from build123d import *

# Parameters (mm, degrees)
SKETCH_R  = 3.302
PAD_DEPTH = 3


with BuildPart() as part:
    # Sketch → Pad (new body)
    with BuildSketch(Plane.XY):
        with BuildLine():
            Line((0, 62.5), (0, 1))
            ThreePointArc((0, 1), (0.292893, 0.292893), (1, 0))
            Line((1, 0), (43.41875, 0))
            ThreePointArc((43.41875, 0), (44.125857, 0.292893), (44.41875, 1))
            Line((44.41875, 1), (44.41875, 24.9))
            ThreePointArc((45.41875, 25.9), (44.711643, 25.607107), (44.41875, 24.9))
            Line((45.41875, 25.9), (125.41865, 25.9))
            ThreePointArc((125.41865, 25.9), (126.125757, 26.192893), (126.41865, 26.9))
            Line((126.41865, 26.9), (126.41865, 62.5))
            ThreePointArc((126.41865, 62.5), (126.125757, 63.207107), (125.41865, 63.5))
            Line((125.41865, 63.5), (1, 63.5))
            ThreePointArc((1, 63.5), (0.292893, 63.207107), (0, 62.5))
        make_face()
        with Locations((22.209375, 12.7)):
            Circle(SKETCH_R, mode=Mode.SUBTRACT)
    extrude(amount=PAD_DEPTH)


solid = part.part
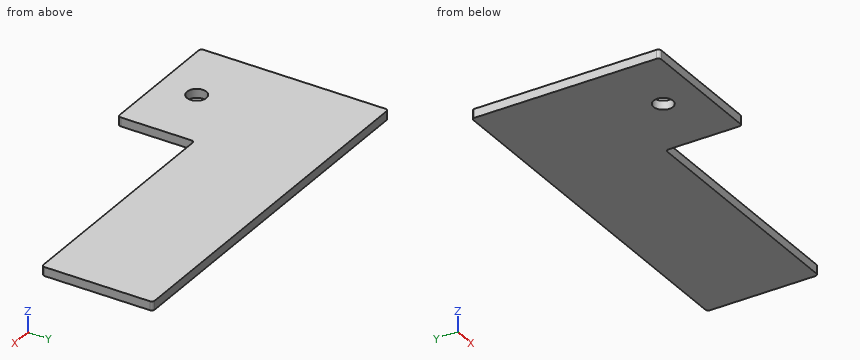
Geometry: final body of the model. Coordinates: model frame, mm. Give positions to 0.01 mm unless a question says otherwise; leave off trailing zeros. Loops run counter-clockwise (first coordinate to the right, second up) from the corner with the lowest first, then second, coordinate; pieces in that order, holes last. Notation, with made-up numbers: M 52,4.25 L 75,4.25 A24 ccw 75,39.25 Z; hole C 84.5,22 d9. An arc over 180 degrees is marked long. Put each result on its own line as item: value. Start each with the question number.
1) Cut plane C-C (x = 61.5). Output: boundary loops of the cut face in (y, z), then the cut area to 3 significant figures.
2) Contact query for a flat-ended pin moving along its axis: pin 1 (1.5 mm diameter, centred on x = 78.5, z = 1.5, fed in from -Y). Output: stop coordinate, or through.
3) Cut plane A-A (y = 12.7). Output: boundary loops of the cut face in (x, z), then the cut area to 3 significant figures.
4) Cut plane B-B (z = 0.95). Output: boundary loops of the cut face in (x, y), then the cut area to 3 significant figures.
5) Ray query, line 1 along Y through (x, z) = (19.5, 2.5); line 2 along X through (y, z) = (20.5, 2.5); line 3 along Y through (x, z) = (83, 0.75). Return the intervals inside material, ascending.
Verdict:
1. outline: M 25.9,0 L 63.5,0 L 63.5,3 L 25.9,3 Z
1. area: 113 mm2
2. pin 1: y = 25.9
3. outline: M 0,0 L 18.91,0 L 18.91,3 L 0,3 Z; M 25.51,0 L 44.42,0 L 44.42,3 L 25.51,3 Z
3. area: 113 mm2
4. outline: M 0,1 A1 ccw 1,0 L 43.42,0 A1 ccw 44.42,1 L 44.42,24.9 A1 cw 45.42,25.9 L 125.42,25.9 A1 ccw 126.42,26.9 L 126.42,62.5 A1 ccw 125.42,63.5 L 1,63.5 A1 ccw 0,62.5 Z; hole C 22.21,12.7 d6.6
4. area: 5,870 mm2
5. line 1: 0 to 10.81, 14.59 to 63.5
5. line 2: 0 to 44.42
5. line 3: 25.9 to 63.5
